Source: CAD feature listing. Evaluate the final solid. Frame: model axes, mm. A direction names the side the tool comes from. Give positions to 0.01 mm unless a question says otherwise; leave off trailing zeros. Loops run counter-clockwise (first coordinate to the right, second up) from the corner with the lowest first, then second, coordinate; pieces in that order, holes last. Notation, with made-up numbers: (53.5, -32.5) -> (83.5, -32.5) arc R16 ccw to (83.5, -17.5) -> close; hole circle Ø9 at (21.25, -22). An arc over 180 degrees is marked (long way). Put each result on its own line as item: value.
```python
from build123d import *

# Parameters (mm, degrees)
BOSS_EXTRUDE1_DEPTH = 3.5
SKETCH3_W           = 13.5
SKETCH3_H           = 6
CUT_EXTRUDE1_DEPTH  = 10
CUT_EXTRUDE2_DEPTH  = 15.5


with BuildPart() as part:
    # Sketch1 → Revolve1 (revolve)
    with BuildSketch(Plane(origin=(0, 0, 0), x_dir=(0, 0, -1), z_dir=(1, 0, 0))):
        Polygon((-32.2, 0), (15.5, 0), (15.5, 10.3), (0, 10.3), (0, 12.56), (-3.2, 12.56), (-3.2, 10.1), (-7.2, 10.1), (-7.2, 3), (-32.2, 3), align=None)
    revolve(axis=Axis((0, 0, -15.5), (0, 0, -1)))

    # Sketch2 → Boss-Extrude1 (add, symmetric)
    with BuildSketch(Plane(origin=(0, 0, 0), x_dir=(1, 0, 0), z_dir=(0, 1, 0))):
        Polygon((-6.75, -7.2), (6.75, -7.2), (4, -19.5), (-4, -19.5), align=None)
    extrude(amount=BOSS_EXTRUDE1_DEPTH, both=True)

    # Sketch3 → Cut-Extrude1 (cut)
    with BuildSketch(Plane(origin=(0, 0, -15.5), x_dir=(-1, 0, 0), z_dir=(0, 0, -1))):
        Rectangle(SKETCH3_W, SKETCH3_H)
    extrude(amount=-CUT_EXTRUDE1_DEPTH, mode=Mode.SUBTRACT)

    # Sketch4 → Cut-Extrude2 (cut)
    with BuildSketch(Plane(origin=(0, 0, -15.5), x_dir=(-1, 0, 0), z_dir=(0, 0, -1))):
        with BuildLine():
            Line((8.6, 5.668333088), (8.6, -5.668333088))
            ThreePointArc((8.6, -5.668333088), (10.3, 0), (8.6, 5.668333088))
        make_face()
    extrude(amount=-CUT_EXTRUDE2_DEPTH, mode=Mode.SUBTRACT)


solid = part.part
```
(1) Section C-C on x = 0. Return loops of the section in (y, z), then the cut area to 3 significant figures.
Calculated:
outline: (-12.56, 0) -> (-10.3, 0) -> (-10.3, -15.5) -> (-3, -15.5) -> (-3, -5.5) -> (3, -5.5) -> (3, -15.5) -> (10.3, -15.5) -> (10.3, 0) -> (12.56, 0) -> (12.56, 3.2) -> (10.1, 3.2) -> (10.1, 7.2) -> (3.5, 7.2) -> (3.5, 19.5) -> (3, 19.5) -> (3, 32.2) -> (-3, 32.2) -> (-3, 19.5) -> (-3.5, 19.5) -> (-3.5, 7.2) -> (-10.1, 7.2) -> (-10.1, 3.2) -> (-12.56, 3.2) -> close
area: 583 mm²
(2) Section A-A on y = 0. Return loops of the section in (x, z).
Calculated:
outline: (-12.56, 0) -> (-8.6, 0) -> (-8.6, -15.5) -> (-6.75, -15.5) -> (-6.75, -5.5) -> (6.75, -5.5) -> (6.75, -15.5) -> (10.3, -15.5) -> (10.3, 0) -> (12.56, 0) -> (12.56, 3.2) -> (10.1, 3.2) -> (10.1, 7.2) -> (6.75, 7.2) -> (4, 19.5) -> (3, 19.5) -> (3, 32.2) -> (-3, 32.2) -> (-3, 19.5) -> (-4, 19.5) -> (-6.75, 7.2) -> (-10.1, 7.2) -> (-10.1, 3.2) -> (-12.56, 3.2) -> close
(3) Reachability of faces 1 (the flat face through (0, 3.5, 13)), 2 (the flat face through (-9, -1, 0)), 3 (the flat face through (3, 2, 19.5)), 4 (the flat face through (-8.6, 0, -8)) from +Z, -Z, +X, -X, +Y, -Y: full face, straight path, thin tool, end or side. Return the list, or none.
Calculated:
face 1: +Z, +X, -X, +Y
face 2: -Z
face 3: +Z
face 4: -Z, -X, +Y, -Y
(4) Section B-B on z = -9. Return loops of the section in (x, y), then the cut area to 3 significant figures.
Calculated:
outline: (-8.6, -5.67) arc R10.3 ccw (long way) to (-8.6, 5.67) -> close; hole (-6.75, -3) -> (6.75, -3) -> (6.75, 3) -> (-6.75, 3) -> close
area: 239 mm²
(5) First-contact query: P1, Ø5, axis at x = 0.5, y = 0, coming from the -Z side; P2, Ø6, axis at x = -2, z = 15.5, coming from the +Y side; P3, Ø10, axis at x = -8.5, y = -3.5, coming from the +Z side. Flat tips, straight axial feed; report the tip coordinate or a pass-through.
Calculated:
P1: stops at z = -5.5
P2: stops at y = 3.5
P3: stops at z = 19.5
(6) Section D-D on z = -3. Return loops of the section in (x, y).
Calculated:
outline: (-8.6, -5.67) arc R10.3 ccw (long way) to (-8.6, 5.67) -> close
(7) Line query: probe 1 along Z at (x, y) = (-9.5, 2.5); probe 2 along Y at (x, z) = (1.5, 15); probe 3 along Z at (x, y) = (-9.5, 5.5). Output: solid intervals per line, ascending. Write a range as from..to.
Calculated:
probe 1: z = 0..7.2
probe 2: y = -3.5..3.5
probe 3: z = 0..3.2
(8) Draft query along Y for faces 5 (the flat face through (0, 3, -11)), 6 (the flat face through (5.394, 0.049, 13.264)), 7 (the cylindrical face through (10.293, 0.369, -7.642)). Return one class per face: released by +Y, released by -Y, zero draft, split by the parting line, or undercut.
Calculated:
face 5: undercut
face 6: zero draft
face 7: split by the parting line
